```python
from build123d import *

# Parameters (mm, degrees)
BOSS_EXTRUDE1_DEPTH = 7.5
CUT_EXTRUDE1_DEPTH  = 2
BOSS_EXTRUDE2_DEPTH = 2
BOSS_EXTRUDE3_DEPTH = 2


with BuildPart() as part:
    # Sketch1 → Boss-Extrude1 (new body)
    # profile 1 of 2: a face of its own
    with BuildSketch(Plane(origin=(0, 0, 0), x_dir=(1, 0, 0), z_dir=(0, 1, 0))):
        Polygon((-5.196152423, -9), (5.196152423, -9), (10.392304845, 0), (5.196152423, 9), (-5.196152423, 9), (-10.392304845, 0), align=None)
        Polygon((4.330127019, -7.5), (8.660254038, 0), (4.330127019, 7.5), (-4.330127019, 7.5), (-8.660254038, 0), (-4.330127019, -7.5), align=None, mode=Mode.SUBTRACT)
    # profile 2 of 2: a face of its own
    with BuildSketch(Plane(origin=(0, 0, 0), x_dir=(1, 0, 0), z_dir=(0, 1, 0))):
        Polygon((-4.330127019, -7.5), (4.330127019, -7.5), (8.660254038, 0), (4.330127019, 7.5), (-4.330127019, 7.5), (-8.660254038, 0), align=None)
    extrude(amount=BOSS_EXTRUDE1_DEPTH)

    # Sketch1_3 → Cut-Extrude1 (cut)
    with BuildSketch(Plane(origin=(0, 0, 0), x_dir=(1, 0, 0), z_dir=(0, 1, 0))):
        Polygon((-4.330127019, -7.5), (4.330127019, -7.5), (8.660254038, 0), (4.330127019, 7.5), (-4.330127019, 7.5), (-8.660254038, 0), align=None)
    extrude(amount=CUT_EXTRUDE1_DEPTH, mode=Mode.SUBTRACT)

    # Sketch4 → Boss-Extrude2 (add)
    with BuildSketch(Plane(origin=(0, 7.5, 0), x_dir=(1, 0, 0), z_dir=(0, 1, 0))):
        Polygon((8.660254038, 0), (4.330127019, 7.5), (-4.330127019, 7.5), (-8.660254038, 0), (-4.330127019, -7.5), (4.330127019, -7.5), align=None)
    extrude(amount=BOSS_EXTRUDE2_DEPTH)

    # Cut-Sweep3: sweep along a path in Sketch7
    with BuildLine(Plane(origin=(0, 9.5, 0), x_dir=(1, 0, 0), z_dir=(0, 1, 0))) as cut_sweep3_path:
        Line((-6.495190528, -3.75), (-3, -1.732050808))
        ThreePointArc((-3, -1.732050808), (-0.803847577, 0.464101615), (0, 3.464101615))
        Line((0, 3.464101615), (0, 7.5))
    # Sketch5 → Cut-Sweep3 (sweep, cut)
    with BuildSketch(Plane(origin=(-6.495190528, 0, 3.75), x_dir=(0.5000000000000006, 0, 0.8660254037844384), z_dir=(-0.8660254037844384, 0, 0.5000000000000006))):
        with BuildLine():
            Line((-4.330127019, 9.5), (4.330127019, 9.5))
            ThreePointArc((4.330127019, 9.5), (3.446243542, 9.133883476), (3.080127019, 8.25))
            ThreePointArc((3.080127019, 8.25), (2.860457105, 7.719669914), (2.330127019, 7.5))
            Line((2.330127019, 7.5), (-2.330127019, 7.5))
            ThreePointArc((-2.330127019, 7.5), (-2.860457105, 7.719669914), (-3.080127019, 8.25))
            ThreePointArc((-3.080127019, 8.25), (-3.446243542, 9.133883476), (-4.330127019, 9.5))
        make_face()
    sweep(path=cut_sweep3_path.line, mode=Mode.SUBTRACT)

    # Sketch8 → Boss-Extrude3 (add)
    with BuildSketch(Plane(origin=(0, 9.5, 0), x_dir=(1, 0, 0), z_dir=(0, 1, 0))):
        with BuildLine():
            Line((-0.834936491, -5.482050808), (-4.330127019, -7.5))
            Line((-4.330127019, -7.5), (4.330127019, -7.5))
            Line((4.330127019, -7.5), (8.660254038, 0))
            Line((8.660254038, 0), (4.330127019, 7.5))
            Line((4.330127019, 7.5), (4.330127019, 3.464101615))
            ThreePointArc((4.330127019, 3.464101615), (2.946152423, -1.700961894), (-0.834936491, -5.482050808))
        make_face()
    extrude(amount=BOSS_EXTRUDE3_DEPTH)


solid = part.part
```
Here's how the part is built. I have some questions about the finished solid (model axes, mm). A direction names the side the tool comes from. Give positions to 0.01 mm unless a question says otherwise; leave off trailing zeros. Write each loop counter-clockwise with the first axis right and the second up, starting at its lowest first coordinate (ties: lowest second). Pieces come first, ordered by that corner, then holes. Notation, with made-up numbers: M -36,-32.75 L 3,-32.75 A22 ccw 3,-24.75 Z; hole C -29,67 d4. An arc over 180 degrees is marked long. Put each result on its own line as item: value. Start each with the question number.
Item 1: If we section it at A-A, the plane y = 8.75: Write out the boundary of the cut face in (x, z).
Item 2: I need wall thicknesses on L1, parallel to Z at x = -0.25, y = 1.25; L2, parallel to Y at x = -5.25, z = 1.5; L3, parallel to Y at x = -5.5, z = -4.75. Which ranges of each line are inside material? Lowest first, please. Write a range as from..to.
Item 3: If we section it at B-B, the plane y = 5: Write out the boundary of the cut face in (x, z), then the cut area to 3 significant figures.
Item 4: Will these pins go through, and if not, where does the flat tip stop? pin 1 (6 mm diameter, centred on x = -4.5, z = 1, fed in from +Y); pin 2 (5 mm diameter, centred on y = 9.5, z = 6.5, fed in from -X); pin 3 (0.6 mm diameter, centred on x = 3, y = 8, fed in from -Z).
Item 5: Thinking about a two-plate mould opening in Z: for faces 1 (the flat face through (0, 2, 0)), 2 (the flat face through (0, 4, 9)), 3 (the cylindrical face through (3.437, 9.124, -5.51)), 4 (the flat face through (-6.526, 0.986, 3.698)), which applies, +Z half, -Z half, draft (parallel to the pull), parting line (faces both ways), or undercut?
Item 6: If we section it at D-D, the plane x = 7.75: Write out the boundary of the cut face in (y, z), then the cut area to 3 significant figures.
Item 7: If we section it at C-C, the plane z = -5.75: Write out the boundary of the cut face in (x, y), then the cut area to 3 significant figures.
Item 8: On a 3-axis mill with a long thin cutter (end or side, diameter ignored), from which of +Z, -Z, +X, -X, +Y, -Y can I reach the whole of each face in a straight line? I mean faces 5 (the cylindrical face through (-3.456, 9.144, -5.51)), 6 (the flat face through (0, 7.5, 0)), 7 (the flat face through (0, 9, 7.5)), 8 (the cylindrical face through (2.98, 10.49, 1.64)). Say none if no direction works.
Values:
1. outline: M -8.66,0 L -4.33,-7.5 L -3.18,-7.5 L -3.18,-3.46 A2.82 ccw -4.59,-1.03 L -8.09,0.99 Z; M -4.9,6.51 L -1.41,4.49 A9.18 cw 3.18,-3.46 L 3.18,-7.5 L 4.33,-7.5 L 8.66,0 L 4.33,7.5 L -4.33,7.5 Z
2. L1: -9..-7.5, 7.5..9
2. L2: 2..7.5
2. L3: 2..9.5
3. outline: M -10.39,0 L -5.2,-9 L 5.2,-9 L 10.39,0 L 5.2,9 L -5.2,9 Z
3. area: 281 mm²
4. pin 1: y = 9.5
4. pin 2: x = -7.51
4. pin 3: z = -7.5
5. face 1: undercut
5. face 2: +Z half
5. face 3: draft
5. face 4: undercut
6. outline: M 0,-4.58 L 7.5,-4.58 L 7.5,-1.58 L 11.5,-1.58 L 11.5,1.58 L 7.5,1.58 L 7.5,4.58 L 0,4.58 L 0,1.58 L 2,1.58 L 2,-1.58 L 0,-1.58 Z
6. area: 75.0 mm²
7. outline: M -7.07,0 L -5.34,0 L -5.34,2 L 5.34,2 L 5.34,0 L 7.07,0 L 7.07,7.5 L 5.34,7.5 L 5.34,11.5 L 4.33,11.5 L 4.33,9.5 A1.25 ccw 3.08,8.25 A0.75 cw 2.33,7.5 L -2.33,7.5 A0.75 cw -3.08,8.25 A1.25 ccw -4.33,9.5 L -5.34,9.5 L -5.34,7.5 L -7.07,7.5 Z
7. area: 95.4 mm²
8. face 5: -Z, +Y
8. face 6: +Y
8. face 7: +Z, +X, -X, +Y
8. face 8: -Z, -X, +Y
